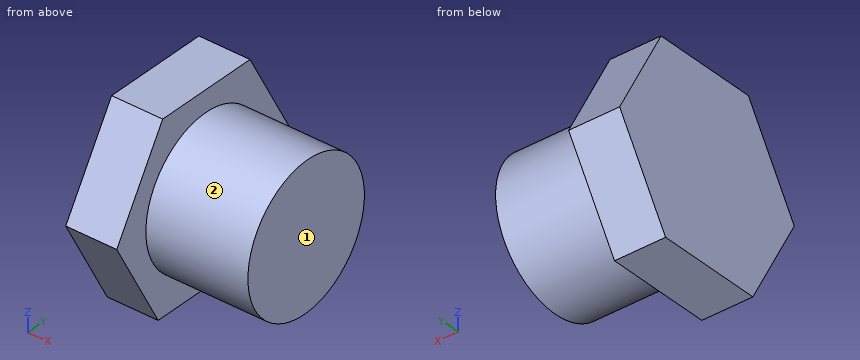
```python
from build123d import *

# Parameters (mm, degrees)
CROQUIS1_R              = 10
SALIENTE_EXTRUIR1_DEPTH = 14
CROQUIS2_R              = 15
SALIENTE_EXTRUIR2_DEPTH = 7
CORTAR_EXTRUIR1_DEPTH   = 30.849623113


with BuildPart() as part:
    # Croquis1 → Saliente-Extruir1 (new body)
    with BuildSketch(Plane(origin=(0, 0, 0), x_dir=(0, 0, -1), z_dir=(1, 0, 0))):
        Circle(CROQUIS1_R)
    extrude(amount=SALIENTE_EXTRUIR1_DEPTH)

    # Croquis2 → Saliente-Extruir2 (add)
    with BuildSketch(Plane.ZY):
        Circle(CROQUIS2_R)
    extrude(amount=SALIENTE_EXTRUIR2_DEPTH)

    # Croquis5 → Cortar-Extruir1 (cut, through all)
    with BuildSketch(Plane.ZY.offset(7)):
        with BuildLine():
            Line((-13.208306062, 7.109194819), (-0.447409717, 14.993326))
            ThreePointArc((-0.447409717, 14.993326), (-7.884131181, 12.760896345), (-13.208306062, 7.109194819))
        make_face()
        with BuildLine():
            Line((-12.760896345, -7.884131181), (-13.208306062, 7.109194819))
            ThreePointArc((-13.208306062, 7.109194819), (-14.993326, -0.447409717), (-12.760896345, -7.884131181))
        make_face()
        with BuildLine():
            Line((0.447409717, -14.993326), (-12.760896345, -7.884131181))
            ThreePointArc((-12.760896345, -7.884131181), (-7.109194819, -13.208306062), (0.447409717, -14.993326))
        make_face()
        with BuildLine():
            ThreePointArc((0.447409717, -14.993326), (7.884131181, -12.760896345), (13.208306062, -7.109194819))
            Line((13.208306062, -7.109194819), (0.447409717, -14.993326))
        make_face()
        with BuildLine():
            ThreePointArc((15, 0), (14.429370138, 4.097960153), (12.760896345, 7.884131181))
            Line((12.760896345, 7.884131181), (13.208306062, -7.109194819))
            ThreePointArc((13.208306062, -7.109194819), (14.545181177, -3.665747473), (15, 0))
        make_face()
        with BuildLine():
            ThreePointArc((12.760896345, 7.884131181), (7.109194819, 13.208306062), (-0.447409717, 14.993326))
            Line((-0.447409717, 14.993326), (12.760896345, 7.884131181))
        make_face()
    extrude(amount=-CORTAR_EXTRUIR1_DEPTH, mode=Mode.SUBTRACT)


solid = part.part
```
Read the model definition and answer for the solid it produces. Units are mm, in the model's axes. Face numbers are marked on the shaded views. A direction names the side the tool comes from. Coordinates: 2 decimals unless noted, no trailing zeros. Loops run counter-clockwise (first coordinate to the right, second up) from the corner with the lowest first, then second, coordinate; pieces in that order, holes last.
(1) Consider line 1 along X through (y, z) = (-9.25, -6); line 2 along Y through (x, z) = (8.25, 0); line 3 along Y through (x, z) = (-1, 1.5). Determine where each line is inside the solid, lowest interval first.
Solution:
line 1: x = -7 to 0
line 2: y = -10 to 10
line 3: y = -14.34 to 13.95
(2) The part is cut by section D-D (x = 7). Determine the outline of the cut face in (y, z).
Solution:
outline: circle Ø20 at (0, 0)
(3) The part is cut by section C-C (z = 5). Determine the outline of the cut face in (x, y), and give its area (3 significant figures).
Solution:
outline: (-7, -12.18) - (0, -12.18) - (0, -8.66) - (14, -8.66) - (14, 8.66) - (0, 8.66) - (0, 12.06) - (-7, 12.06) - close
area: 412 mm2
(4) The part is cut by section A-A (x = -4). Determine the outline of the cut face in (y, z).
Solution:
outline: (-14.99, 0.45) - (-7.88, -12.76) - (7.11, -13.21) - (14.99, -0.45) - (7.88, 12.76) - (-7.11, 13.21) - close
(5) The part is cut by section B-B (y = 0). Determine the outline of the cut face in (x, z), and give its area (3 significant figures).
Solution:
outline: (-7, -13) - (0, -13) - (0, -10) - (14, -10) - (14, 10) - (0, 10) - (0, 13) - (-7, 13) - close
area: 462 mm2
(6) A tool of negligible diameter and unlimited length cuts with its end or side. For the marked faces 1 and 2, from which of +Z, -Z, +X, -X, +Y, -Y can it reach the whole face along a straight path? Write none if from no direction.
Solution:
face 1: +Z, -Z, +X, +Y, -Y
face 2: +X
(7) Flat-ended cylindrical pins translate along their axes: pin 1 Ø1.5 at (x, z) = (8, -3) entering from +Y; pin 2 Ø10 at (x, y) = (10.5, -9.5) entering from -Z; pin 3 Ø4 at (x, z) = (7, 2) entering from +Y. Find the tip coordinate at first contact, or state that the pin passes through.
Solution:
pin 1: stops at y = 9.74
pin 2: stops at z = -8.93
pin 3: stops at y = 10
